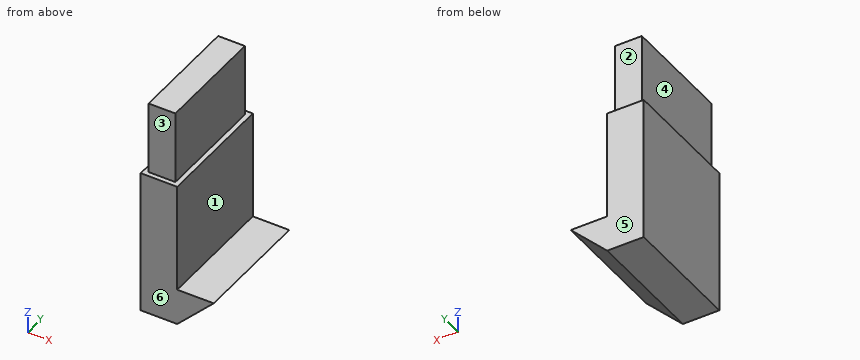
```python
from build123d import *

# Parameters (mm, degrees)
BOSS_EXTRUDE1_DEPTH = 5
SKETCH2_W           = 1.1
SKETCH2_H           = 4.6
BOSS_EXTRUDE2_DEPTH = 3


with BuildPart() as part:
    # Sketch1 → Boss-Extrude1 (new body)
    with BuildSketch(Plane(origin=(0, 0, 0), x_dir=(1, 0, 0), z_dir=(0, 1, 0))):
        Polygon((2.25, 1.5), (0.75, 3), (-0.75, 3), (-0.75, -3), (0.75, -3), (0.75, 1.5), align=None)
    extrude(amount=BOSS_EXTRUDE1_DEPTH)

    # Sketch2 → Boss-Extrude2 (add)
    with BuildSketch(Plane.XY.offset(3)):
        with Locations((0, 2.5)):
            Rectangle(SKETCH2_W, SKETCH2_H)
    extrude(amount=BOSS_EXTRUDE2_DEPTH)


solid = part.part
```
Design review of the part built by this model. Coordinates are the model's own, in mm. Face numbers are marked on the shaded views. A direction names the side the tool comes from. Round coordinates to 2 decimals unless told otherwise and drop trailing zeros. Write each loop counter-clockwise with the first axis right and the second up, starting at its lowest first coordinate (ties: lowest second). Pieces come first, ordered by that corner, then holes.
Item 1: Clearance check with flat-ended pins moving along their axes: pin 1 Ø0.8 at (x, y) = (1.5, 2) entering from +Z; pin 2 Ø1.2 at (x, z) = (-0.5, 5) entering from +Y; pin 3 Ø1 at (x, z) = (1, 1) entering from -Y; pin 4 Ø2 at (y, z) = (3.5, 0) entering from +X. State where each tip first meets the part, or that it passes through.
Item 2: We need section D-D on x = 1.6. Write out the cut boundary in (y, z).
Item 3: We need section B-B on y = 3.9. Write out the cut boundary in (x, z), and give its area (3 significant figures).
Item 4: For probe 1 along X at (y, z) = (4.05, -0.25); probe 2 along Z at (x, y) = (-0.6, 1.05); probe 3 along X at (y, z) = (2.7, 3.75), list the stretches that pass through material, from the lowest coordinate up.
Item 5: We need section C-C on z = 3.25. Write out the cut boundary in (x, y), and give its area (3 significant figures).
Item 6: The part is to be moulded in two halves that separate along Y. For the marked faces 4, 5 and 6, say which applies: +Y half, -Y half, draft (parallel to the pull), parting line (faces both ways), or undercut.
Item 7: For the marked faces 1, 2 and 3, list the 3-axis set-ups (+Z, -Z, +X, -X, +Y, -Y) from which the entire face can be reached by the end or side of a thin tool; tool diameter is ignored.
Item 8: We need section A-A on x = 0. Write out the cut boundary in (y, z), and give its area (3 significant figures).
Returned:
1. pin 1: stops at z = -1.5
1. pin 2: stops at y = 4.8
1. pin 3: stops at y = 0
1. pin 4: stops at x = 0.75
2. outline: (0, -2.15) - (5, -2.15) - (5, -1.5) - (0, -1.5) - close
3. outline: (-0.75, -3) - (0.75, -3) - (2.25, -1.5) - (0.75, -1.5) - (0.75, 3) - (0.55, 3) - (0.55, 6) - (-0.55, 6) - (-0.55, 3) - (-0.75, 3) - close
3. area: 13.4 mm2
4. probe 1: x = -0.75 to 0.75
4. probe 2: z = -3 to 3
4. probe 3: x = -0.55 to 0.55
5. outline: (-0.55, 0.2) - (0.55, 0.2) - (0.55, 4.8) - (-0.55, 4.8) - close
5. area: 5.06 mm2
6. face 4: draft
6. face 5: +Y half
6. face 6: -Y half
7. face 1: +Z, +X, +Y, -Y
7. face 2: +Z, +X, -X, +Y
7. face 3: +Z, +X, -X, -Y
8. outline: (0, -3) - (5, -3) - (5, 3) - (4.8, 3) - (4.8, 6) - (0.2, 6) - (0.2, 3) - (0, 3) - close
8. area: 43.8 mm2
